Geometry: final body of the model. Coordinates: model frame, mm. A direction names the side the tool comes from. Round coordinates to 2 decimals unless told otherwise and drop trailing zeros. Write each loop counter-clockwise with the first axis right and the second up, starting at its lowest first coordinate (ties: lowest second). Pieces come first, ordered by that corner, then holes. Notation, with made-up numbers: M 60,85.5 L 118,85.5 A17 cw 118,110.5 Z; hole C 49.25,67 d2. An arc over 180 degrees is marked long. Answer as CSV lines item,"result". Start each with the question number.
Q1. First-contact query: pin 1 (6 mm diameter, centred on x = -23.57, z = 23.57, fed in from -Y); pin 2 (3 mm diameter, centred on y = 26.5, z = 9.5, fed in from +X); pin 3 (1.5 mm diameter, centred on x = -7, z = -18, fed in from +Y). Flat tips, straight axial feed; report the tip coordinate or a pass-through.
Q2. Ray query, probe 1 along Z at (x, y) = (0, 35); probe 2 along X at (y, z) = (77.9, -23.57). Return the intervals inside material, ascending.
Q3. Section query C-C on y = 49.5. Output: boundary loops of the cut face in (x, z), and give its area (3 significant figures).
Q4. Section query B-B on z = 23.57. Output: boundary loops of the cut face in (x, y).
Q5. Reachability of faces 4 (the flat face through (21, 76, 20)), 5 (the flat face through (-0.4, 81, -19.2)), 6 (the cylindrical face through (13.01, 37.47, 25.02)) from +Z, -Z, +X, -X, +Y, -Y: full face, straight path, thin tool, end or side. Return the list, or none.
Q6. Section query A-A on x = -22.5. Output: boundary loops of the cut face in (y, z), and give its area (3 significant figures).
Q7. Mould query, pull axis X, two halves, no side actions, for faces 1 (the cylindrical face through (-23.9, 78.54, -26.05)), 2 (the flat face through (-21, 76, 21)), 3 (the flat face through (28.2, 78, 0)). Classes: pulls with the +X half, pulls with the -X half, needs draft (parallel to the pull), parting line crosses it, or undercut.
```python
from build123d import *

# Parameters (mm, degrees)
SKETCH1_R           = 28.2
BOSS_EXTRUDE1_DEPTH = 76
BOSS_EXTRUDE3_DEPTH = 5
SKETCH4_R           = 2.5
CUT_EXTRUDE1_DEPTH  = 5
SKETCH5_R           = 19.05
BOSS_EXTRUDE4_DEPTH = 1.6
FILLET1_R           = 1
SKETCH7_R           = 3.2
CUT_EXTRUDE3_DEPTH  = 83.6


with BuildPart() as part:
    # Sketch1 → Boss-Extrude1 (new body)
    with BuildSketch(Plane(origin=(0, 0, 0), x_dir=(1, 0, 0), z_dir=(0, 1, 0))):
        Circle(SKETCH1_R)
    extrude(amount=BOSS_EXTRUDE1_DEPTH)

    # Sketch2 → Boss-Extrude3 (add)
    with BuildSketch(Plane(origin=(0, 76, 0), x_dir=(1, 0, 0), z_dir=(0, 1, 0))):
        with BuildLine():
            Line((-21.2, -28.2), (21.2, -28.2))
            ThreePointArc((21.2, -28.2), (26.149747468, -26.149747468), (28.2, -21.2))
            Line((28.2, -21.2), (28.2, 21.2))
            ThreePointArc((28.2, 21.2), (26.149747468, 26.149747468), (21.2, 28.2))
            Line((21.2, 28.2), (-21.2, 28.2))
            ThreePointArc((-21.2, 28.2), (-26.149747468, 26.149747468), (-28.2, 21.2))
            Line((-28.2, 21.2), (-28.2, -21.2))
            ThreePointArc((-28.2, -21.2), (-26.149747468, -26.149747468), (-21.2, -28.2))
        make_face()
    extrude(amount=BOSS_EXTRUDE3_DEPTH)

    # Sketch4 → Cut-Extrude1 (cut)
    with BuildSketch(Plane(origin=(0, 81, 0), x_dir=(1, 0, 0), z_dir=(0, 1, 0))):
        with Locations((-23.57, 23.57)):
            Circle(SKETCH4_R)
        with Locations((23.57, 23.57)):
            Circle(SKETCH4_R)
        with Locations((-23.57, -23.57)):
            Circle(SKETCH4_R)
        with Locations((23.57, -23.57)):
            Circle(SKETCH4_R)
    extrude(amount=-CUT_EXTRUDE1_DEPTH, mode=Mode.SUBTRACT)

    # Sketch5 → Boss-Extrude4 (add)
    with BuildSketch(Plane(origin=(0, 81, 0), x_dir=(1, 0, 0), z_dir=(0, 1, 0))):
        Circle(SKETCH5_R)
    extrude(amount=BOSS_EXTRUDE4_DEPTH)

    # Fillet1
    fillet1_edges = [part.edges().sort_by_distance(p)[0] for p in [
        (-19.05, 82.6, 0),
    ]]
    fillet(fillet1_edges, radius=FILLET1_R)

    # Sketch7 → Cut-Extrude3 (cut, through all)
    with BuildSketch(Plane(origin=(0, 82.6, 0), x_dir=(1, 0, 0), z_dir=(0, 1, 0))):
        Circle(SKETCH7_R)
    extrude(amount=-CUT_EXTRUDE3_DEPTH, mode=Mode.SUBTRACT)


solid = part.part
```
Entries:
1,pin 1,"stops at y = 76"
1,pin 2,"stops at x = 27.04"
1,pin 3,"stops at y = 82.46"
2,probe 1,"z = -28.2 to -3.2, 3.2 to 28.2"
2,probe 2,"x = -27.79 to -26.07, -21.07 to 21.07, 26.07 to 27.79"
3,outline,"C 0,0 d56.4; hole C 0,0 d6.4"
3,area,"2,470 mm^2"
4,outline,"M -27.79,76 L -26.07,76 L -26.07,81 L -27.79,81 Z; M -21.07,76 L -15.48,76 L -15.48,0 L 15.48,0 L 15.48,76 L 21.07,76 L 21.07,81 L -21.07,81 Z; M 26.07,76 L 27.79,76 L 27.79,81 L 26.07,81 Z"
5,face 4,"+Z, +X, -Y"
5,face 5,"+Y"
5,face 6,"-Y"
6,outline,"M 0,-17 L 76,-17 L 76,-21.31 L 81,-21.31 L 81,21.31 L 76,21.31 L 76,17 L 0,17 Z; M 76,-28.08 L 81,-28.08 L 81,-25.83 L 76,-25.83 Z; M 76,25.83 L 81,25.83 L 81,28.08 L 76,28.08 Z"
6,area,"2,820 mm^2"
7,face 1,"undercut"
7,face 2,"needs draft"
7,face 3,"pulls with the +X half"
